Work out the finished part from the listing and answer in its coordinate system (mm). Round coordinates to 2 decimals unless told otherwise and drop trailing zeros. Write each loop counter-clockwise with the first axis right and the second up, starting at its lowest first coordinate (ties: lowest second). Pieces come first, ordered by that corner, then holes. Notation, with made-up numbers: (0, 8) - (47, 8) arc R19 cw to (47, 27) - close; hole circle Ø6 at (5.25, 79.5). An arc over 180 degrees is marked (long way). Answer as a JSON object with one key per item and string values.
```python
from build123d import *

# Parameters (mm, degrees)
BOSS_EXTRUDE1_DEPTH = 10


with BuildPart() as part:
    # Sketch1 → Boss-Extrude1 (new, symmetric)
    with BuildSketch(Plane(origin=(0, 0, 0), x_dir=(0, 0, -1), z_dir=(1, 0, 0))):
        with BuildLine():
            Line((-99.315402363, -30.342537444), (58.309854952, 60.662447298))
            ThreePointArc((58.309854952, 60.662447298), (66.611935212, 60.127841079), (69.313108369, 52.259295849))
            Line((69.313108369, 52.259295849), (47.967793309, -28.886485338))
            ThreePointArc((47.967793309, -28.886485338), (44.402545097, -34.262116945), (38.296788753, -36.342537444))
            Line((38.296788753, -36.342537444), (-110.536380347, -36.342537444))
            ThreePointArc((-110.536380347, -36.342537444), (-117.053891299, -31.896368093), (-115.29198584, -24.205980582))
            Line((-115.29198584, -24.205980582), (-102.51761164, -12.379014435))
            ThreePointArc((-102.51761164, -12.379014435), (-98.726134685, -12.366723669), (-98.713843919, -16.158200625))
            Line((-98.713843919, -16.158200625), (-106.051782293, -22.951922758))
            Line((-106.051782293, -22.951922758), (-99.315402363, -30.342537444))
        make_face()
        with BuildLine():
            Line((52.017451593, 50.914073792), (30.709901091, -30.088142654))
            Line((30.709901091, -30.088142654), (41.447586102, -30.088142654))
            Line((41.447586102, -30.088142654), (62.847268014, 51.26431811))
            ThreePointArc((62.847268014, 51.26431811), (61.766798752, 54.411736202), (58.445966648, 54.62557869))
            Line((58.445966648, 54.62557869), (52.017451593, 50.914073792))
        make_face(mode=Mode.SUBTRACT)
        with BuildLine():
            Line((15.709901091, -30.088142654), (26.447586102, -30.088142654))
            Line((26.447586102, -30.088142654), (45.161270866, 41.053302896))
            ThreePointArc((45.161270866, 41.053302896), (44.080801604, 44.200720988), (40.7599695, 44.414563475))
            Line((40.7599695, 44.414563475), (34.331454445, 40.703058578))
            Line((34.331454445, 40.703058578), (15.709901091, -30.088142654))
        make_face(mode=Mode.SUBTRACT)
        with BuildLine():
            Line((0.709901092, -30.088142654), (11.447586102, -30.088142654))
            Line((11.447586102, -30.088142654), (27.475273718, 30.842287682))
            ThreePointArc((27.475273718, 30.842287682), (26.394804456, 33.989705774), (23.073972352, 34.203548261))
            Line((23.073972352, 34.203548261), (16.645457297, 30.492043364))
            Line((16.645457297, 30.492043364), (0.709901092, -30.088142654))
        make_face(mode=Mode.SUBTRACT)
        with BuildLine():
            Line((-14.290098908, -30.088142654), (-3.552413898, -30.088142654))
            Line((-3.552413898, -30.088142654), (9.789276571, 20.631272467))
            ThreePointArc((9.789276571, 20.631272467), (8.708807308, 23.778690559), (5.387975204, 23.992533047))
            Line((5.387975204, 23.992533047), (-1.040539851, 20.28102815))
            Line((-1.040539851, 20.28102815), (-14.290098908, -30.088142654))
        make_face(mode=Mode.SUBTRACT)
        with BuildLine():
            Line((-29.290098908, -30.088142654), (-18.552413898, -30.088142654))
            Line((-18.552413898, -30.088142654), (-7.896720577, 10.420257253))
            ThreePointArc((-7.896720577, 10.420257253), (-8.97718984, 13.567675345), (-12.298021944, 13.781517833))
            Line((-12.298021944, 13.781517833), (-18.726536999, 10.070012936))
            Line((-18.726536999, 10.070012936), (-29.290098908, -30.088142654))
        make_face(mode=Mode.SUBTRACT)
        with BuildLine():
            Line((-44.290098908, -30.088142654), (-33.552413898, -30.088142654))
            Line((-33.552413898, -30.088142654), (-25.582717725, 0.209242039))
            ThreePointArc((-25.582717725, 0.209242039), (-26.663186988, 3.356660131), (-29.984019092, 3.570502619))
            Line((-29.984019092, 3.570502619), (-36.412534146, -0.141002279))
            Line((-36.412534146, -0.141002279), (-44.290098908, -30.088142654))
        make_face(mode=Mode.SUBTRACT)
        with BuildLine():
            Line((-59.290098908, -30.088142654), (-48.552413898, -30.088142654))
            Line((-48.552413898, -30.088142654), (-43.268714873, -10.001773175))
            ThreePointArc((-43.268714873, -10.001773175), (-44.349184136, -6.854355083), (-47.67001624, -6.640512596))
            Line((-47.67001624, -6.640512596), (-54.098531294, -10.352017493))
            Line((-54.098531294, -10.352017493), (-59.290098908, -30.088142654))
        make_face(mode=Mode.SUBTRACT)
        with BuildLine():
            Line((-74.290098908, -30.088142654), (-63.552413898, -30.088142654))
            Line((-63.552413898, -30.088142654), (-60.954712021, -20.212788389))
            ThreePointArc((-60.954712021, -20.212788389), (-62.035181283, -17.065370297), (-65.356013388, -16.85152781))
            Line((-65.356013388, -16.85152781), (-71.784528442, -20.563032707))
            Line((-71.784528442, -20.563032707), (-74.290098908, -30.088142654))
        make_face(mode=Mode.SUBTRACT)
    extrude(amount=BOSS_EXTRUDE1_DEPTH, both=True)


solid = part.part
```
Item 1: A cutting plane is placed at B-B (x = 3). Give the number of separate pieces and of enclosed holes in the cut face, and give its area (3 significant figures).
Results found:
{"separate pieces": "1", "enclosed holes": "8", "area": "4,310 mm²"}
Item 2: A cutting plane is placed at A-A (y = -4.5). Write down the section's boundary in (x, z).
Results found:
{"outline": "(-10, -54.38) - (10, -54.38) - (10, -48.18) - (-10, -48.18) - close; (-10, -37.44) - (10, -37.44) - (10, -33.18) - (-10, -33.18) - close; (-10, -22.44) - (10, -22.44) - (10, -18.18) - (-10, -18.18) - close; (-10, -7.44) - (10, -7.44) - (10, -3.18) - (-10, -3.18) - close; (-10, 7.56) - (10, 7.56) - (10, 11.82) - (-10, 11.82) - close; (-10, 22.56) - (10, 22.56) - (10, 26.82) - (-10, 26.82) - close; (-10, 37.56) - (10, 37.56) - (10, 54.55) - (-10, 54.55) - close"}
Item 3: Consider line 1 along Z through (x, y) = (2.25, 40.5); line 2 along Z through (x, y) = (4.5, 17); line 3 along Z through (x, y) = (6, 38). Determine where each line is inside the solid, lowest interval first.
Results found:
{"line 1": "-66.22 to -60.02, -49.28 to -45.02, -34.28 to -23.39", "line 2": "-60.04 to -53.83, -43.1 to -38.83, -28.1 to -23.83, -13.1 to -8.83, 1.9 to 17.32", "line 3": "-65.56 to -59.36, -48.62 to -44.36, -33.62 to -19.06"}
Item 4: Determine the mould class of faces 1 (the flat face through (10, -5, 10)), 2 (the flat face through (0, -36.343, 35)), 3 (the flat face through (0.14, -9.728, 23.934)) for opening direction Y: pulls with the +Y half, pulls with the -Y half, needs draft (parallel to the pull), parting line crosses it, or undercut.
Results found:
{"face 1": "needs draft", "face 2": "pulls with the -Y half", "face 3": "undercut"}
Item 5: A cutting plane is placed at D-D (z = 95). Write down the section's boundary in (x, y).
Results found:
{"outline": "(-10, -36.34) - (10, -36.34) - (10, -27.85) - (-10, -27.85) - close"}
Item 6: A cutting plane is placed at C-C (y = 36.5). Write down the section's boundary in (x, z), and give its area (3 significant figures).
Results found:
{"outline": "(-10, -65.17) - (10, -65.17) - (10, -58.96) - (-10, -58.96) - close; (-10, -48.23) - (10, -48.23) - (10, -43.96) - (-10, -43.96) - close; (-10, -33.23) - (10, -33.23) - (10, -16.46) - (-10, -16.46) - close", "area": "545 mm²"}
Item 7: Each of these flat-tipped pins is pushed along its axis until it touches: P1, Ø8.5, axis at x = 1, z = 23.5, coming from the +Y side; P2, Ø5.5, axis at x = 0.5, z = 51.5, coming from the +Y side; P3, Ø12, axis at x = -4.5, z = 41.5, coming from the +Y side. Where does it stop, or does it pass through?
Results found:
{"P1": "y = 15.88", "P2": "y = -1.15", "P3": "y = 6.5"}
